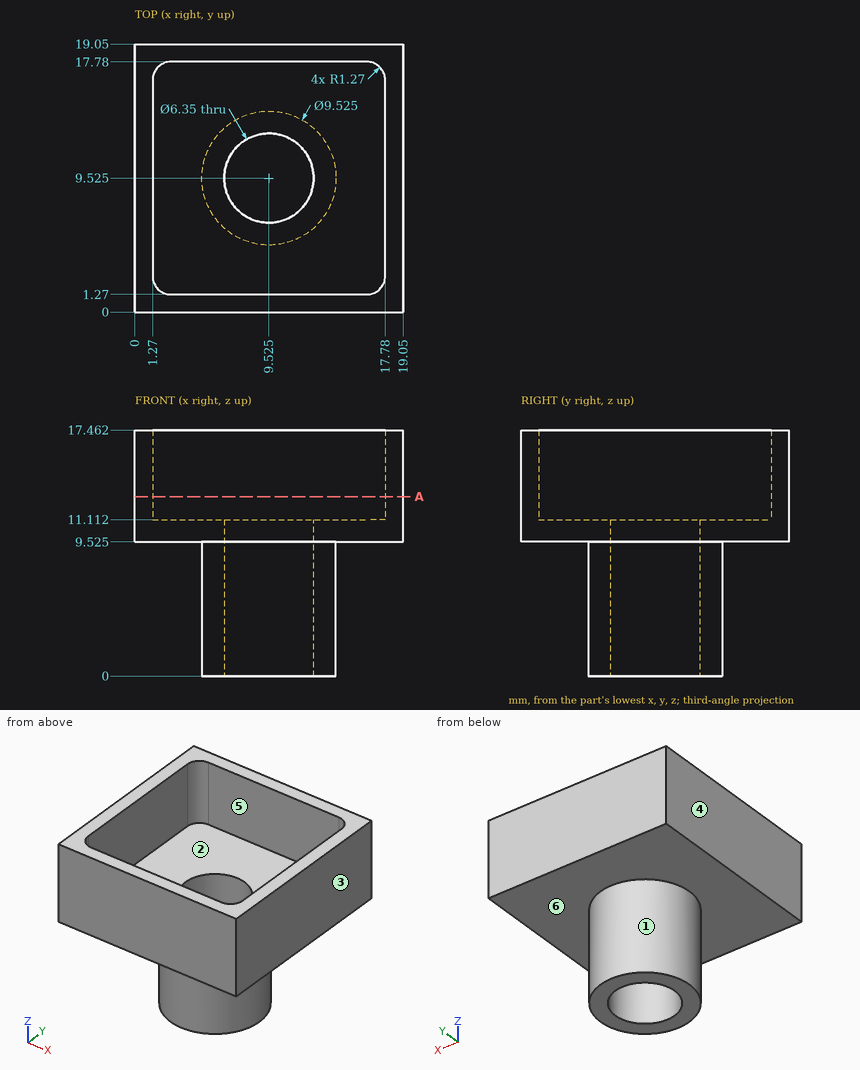
The figure shows three views and two pictorial views of one solid part (mm, origin at its lowest corner). Answer the questions. A direction names the side the tool comes from. Give positions to 0.01 mm unless a question says otherwise; leave off trailing zeros. Order: outer loops, then holes, each group sorted by start corner. A loop starts at its lowest first (then second) coordinate and runs counter-clockwise, first axis right, second up. Notation, with made-up numbers: M 44,21.25 L 71,21.25 A22 ccw 71,32.25 Z; hole C -36.75,49 d4. An arc over 180 degrees is marked long. Return JSON: item names as keys, results as strings.
Q1. The mould has two halves that part along X. Classify the marked faces 4, 5 and 6: pulls with the +X half, pulls with the -X half, needs draft (parallel to the pull), parting line crosses it, or undercut.
Answer below:
{"face 4": "pulls with the -X half", "face 5": "undercut", "face 6": "needs draft"}
Q2. Which of the six approach directions +Z, -Z, +X, -X, +Y, -Y give full straight-line access (tool end or side, diameter ignored) to the marked faces 1, 2 and 3?
Answer below:
{"face 1": "-Z", "face 2": "+Z", "face 3": "+Z, -Z, +X, +Y, -Y"}
Q3. Find section A-A, the plane z = 12.75. Write down the section's boundary in (x, y).
Answer below:
{"outline": "M 0,0 L 19.05,0 L 19.05,19.05 L 0,19.05 Z; hole M 1.27,2.54 A1.27 ccw 2.54,1.27 L 16.51,1.27 A1.27 ccw 17.78,2.54 L 17.78,16.51 A1.27 ccw 16.51,17.78 L 2.54,17.78 A1.27 ccw 1.27,16.51 Z"}
Q4. Each of these flat-tipped pins is pushed along its axis until it touches: pin 1 (5 mm diameter, centred on x = 7.5, y = 12, fed in from +Z); pin 2 (4 mm diameter, centred on x = 16.5, z = 5.5, fed in from -Y). Where does it stop, or does it pass through?
Answer below:
{"pin 1": "stops at z = 11.11", "pin 2": "passes through"}
Q5. Find the intervals of material crossed by line 1 along X through (y, z) = (15, 11.75); line 2 along Z through (x, y) = (5.5, 15) (1 decimal), in increasing order. Write a range as [from, to].
Answer below:
{"line 1": "x = [0, 1.27], [17.78, 19.05]", "line 2": "z = [9.5, 11.1]"}
